Verification items for the finished model (mm, model axes). A direction names the side the tool comes from. Round coordinates to 2 decimals unless told otherwise and drop trailing zeros. Write each loop counter-clockwise with the first axis right and the second up, starting at its lowest first coordinate (ties: lowest second). Pieces come first, ordered by that corner, then holes. Notation, with made-up numbers: (-18, 33) - (-4, 33) arc R11 cw to (-4, 48) - close; hole circle Ø5 at (13.25, 3.25). An arc over 180 degrees is marked (long way). Answer as a JSON object with one key per item and string values.
```python
from build123d import *

# Parameters (mm, degrees)
F1_DEPTH = 50
F0_R     = 15
F2_DEPTH = 30
F3_R     = 10
F4_DEPTH = 42.2


with BuildPart() as f1:
    # F0 (on Front) → F1 (new body)
    with BuildSketch(Plane.XZ):
        with BuildLine():
            ThreePointArc((-4, -19.5959179423), (-12.6491106407, 15.4919333848), (20, 0))
            ThreePointArc((20, 0), (15.4919333848, -12.6491106407), (4, -19.5959179423))
            Line((4, -19.5959179423), (4, -25))
            Line((4, -25), (16.5831239518, -25))
            ThreePointArc((16.5831239518, -25), (20.3783390562, -22.0164324383), (23.6458608502, -18.4627534418))
            ThreePointArc((23.6458608502, -18.4627534418), (28.36702157, -9.7627909558), (30, 0))
            ThreePointArc((30, 0), (26.4338203685, 14.1863716546), (16.5831239518, 25))
            Line((16.5831239518, 25), (-16.5831239518, 25))
            ThreePointArc((-16.5831239518, 25), (-29.6115777819, 4.8119082768), (-23.6458608502, -18.4627534418))
            ThreePointArc((-23.6458608502, -18.4627534418), (-20.3783390562, -22.0164324383), (-16.5831239518, -25))
            Line((-16.5831239518, -25), (-4, -25))
            Line((-4, -25), (-4, -19.5959179423))
        make_face()
        with BuildLine():
            ThreePointArc((16.5831239518, 25), (0, 30), (-16.5831239518, 25))
            Line((-16.5831239518, 25), (16.5831239518, 25))
        make_face()
        with BuildLine():
            Line((16.5831239518, -57.5959179423), (16.5831239518, -25))
            ThreePointArc((16.5831239518, -25), (10.5600439971, -28.079983454), (4, -29.7321374946))
            Line((4, -29.7321374946), (4, -57.5959179423))
            Line((4, -57.5959179423), (16.5831239518, -57.5959179423))
        make_face()
        with BuildLine():
            Line((16.5831239518, -25), (4, -25))
            Line((4, -25), (4, -29.7321374946))
            ThreePointArc((4, -29.7321374946), (10.5600439971, -28.079983454), (16.5831239518, -25))
        make_face()
        with BuildLine():
            ThreePointArc((-4, -29.7321374946), (-10.5600439971, -28.079983454), (-16.5831239518, -25))
            Line((-16.5831239518, -25), (-16.5831239518, -57.5959179423))
            Line((-16.5831239518, -57.5959179423), (-4, -57.5959179423))
            Line((-4, -57.5959179423), (-4, -29.7321374946))
        make_face()
        with BuildLine():
            Line((-4, -29.7321374946), (-4, -25))
            Line((-4, -25), (-16.5831239518, -25))
            ThreePointArc((-16.5831239518, -25), (-10.5600439971, -28.079983454), (-4, -29.7321374946))
        make_face()
    extrude(amount=F1_DEPTH)

    # F0 (on Front) → F2 (join)
    with BuildSketch(Plane.XZ):
        with BuildLine():
            Line((-50, -25), (-23.6458608502, -18.4627534418))
            ThreePointArc((-23.6458608502, -18.4627534418), (-29.6115777819, 4.8119082768), (-16.5831239518, 25))
            Line((-16.5831239518, 25), (-85, 25))
            Line((-85, 25), (-85, -25))
            Line((-85, -25), (-50, -25))
        make_face()
        with Locations((-58.52034688, 0)):
            Circle(F0_R, mode=Mode.SUBTRACT)
        with BuildLine():
            ThreePointArc((30, 0), (28.36702157, -9.7627909558), (23.6458608502, -18.4627534418))
            Line((23.6458608502, -18.4627534418), (50, -25))
            Line((50, -25), (85, -25))
            Line((85, -25), (85, 25))
            Line((85, 25), (16.5831239518, 25))
            ThreePointArc((16.5831239518, 25), (26.4338203685, 14.1863716546), (30, 0))
        make_face()
        with Locations((58.52034688, 0)):
            Circle(F0_R, mode=Mode.SUBTRACT)
    extrude(amount=F2_DEPTH)

    # F3 (on face) → F4 (cut)
    with BuildSketch(Plane(origin=(-16.5831239518, 0, 0), x_dir=(0, -1, 0), z_dir=(-1, 0, 0))):
        with Locations((25, -43)):
            Circle(F3_R)
    extrude(amount=-F4_DEPTH, mode=Mode.SUBTRACT)


solid = f1.part
```
1. Material ranges on probe 1 along X at (y, z) = (-34, -35); probe 2 along X at (y, z) = (-32, 7) (3 decimals); probe 3 along Y at (x, z) = (-59.5, -19), recorded low to high. Write a range as from..to.
Completed:
{"probe 1": "x = -16.58..-4, 4..16.58", "probe 2": "x = -29.172..-18.735, 18.735..29.172", "probe 3": "y = -30..0"}
2. Cross-section at D-D (z = 7). Record the boundary of the cut face in (x, y) (3 decimals).
Completed:
{"outline": "(-85, -30) - (-71.787, -30) - (-71.787, 0) - (-85, 0) - close; (-45.254, -30) - (-29.172, -30) - (-29.172, -50) - (-18.735, -50) - (-18.735, 0) - (-45.254, 0) - close; (18.735, -50) - (29.172, -50) - (29.172, -30) - (45.254, -30) - (45.254, 0) - (18.735, 0) - close; (71.787, -30) - (85, -30) - (85, 0) - (71.787, 0) - close"}
3. Cross-section at C-C (x = 0). Record the boundary of the cut face in (y, z).
Completed:
{"outline": "(-50, 20) - (0, 20) - (0, 30) - (-50, 30) - close"}
4. Access from +Z, -Z, +X, -X, +Y, -Y to the whole of each face (thin tool, end or side, straight path). Record for faces 1 (the face through (-68, -15, -25)), 2 (the face through (-85, -15, 0)), 3 (the face through (16.583, -19, -34)), 4 (the face through (-37.007, -14.79, -21.777)), 5 (the face through (51, -15, 25)).
Completed:
{"face 1": "-Z, -X, +Y, -Y", "face 2": "+Z, -Z, -X, +Y, -Y", "face 3": "-Z, +X, +Y, -Y", "face 4": "-Z, +Y, -Y", "face 5": "+Z, +X, +Y, -Y"}
5. Go/stop test with flat-tipped pins: pin 1 (5 mm diameter, centred on y = -15, z = -34.5, fed in from +X); pin 2 (9 mm diameter, centred on x = -66, y = -21, fed in from -Z); pin 3 (12 mm diameter, centred on y = -40, z = 10.5, fed in from -X). Record where each tip stops, or that it passes through.
Completed:
{"pin 1": "stops at x = 16.58", "pin 2": "stops at z = -25", "pin 3": "stops at x = -29.66"}
6. Cross-section at A-A (y = -25). Record the boundary of the cut face in (x, z).
Completed:
{"outline": "(-85, -25) - (-50, -25) - (-23.65, -18.46) arc R30 ccw to (-16.58, -25) - (-16.58, -33) - (-4, -33) - (-4, -19.6) arc R20 cw (long way) to (4, -19.6) - (4, -33) - (16.58, -33) - (16.58, -25) arc R30 ccw to (23.65, -18.46) - (50, -25) - (85, -25) - (85, 25) - (16.58, 25) arc R30 ccw to (-16.58, 25) - (-85, 25) - close; (-16.58, -57.6) - (-4, -57.6) - (-4, -53) - (-16.58, -53) - close; (4, -57.6) - (16.58, -57.6) - (16.58, -53) - (4, -53) - close; hole circle Ø30 at (-58.52, 0); hole circle Ø30 at (58.52, 0)"}
7. Cross-section at B-B (z = -43). Record the boundary of the cut face in (x, y).
Completed:
{"outline": "(-16.58, -50) - (-4, -50) - (-4, -35) - (-16.58, -35) - close; (-16.58, -15) - (-4, -15) - (-4, 0) - (-16.58, 0) - close; (4, -50) - (16.58, -50) - (16.58, -35) - (4, -35) - close; (4, -15) - (16.58, -15) - (16.58, 0) - (4, 0) - close"}
8. Mould release check, pull along Z, two halves, no side actions. Record for faces 6 (the face through (43.535, -14.79, 0.66)), 7 (the face through (-50, -15, 25)), 8 (the face through (-44, -30, 6)), 9 (the face through (-70.42, -14.79, -9.13)): released by +Z, released by -Z, zero draft, split by the parting line, or undercut.
Completed:
{"face 6": "undercut", "face 7": "released by +Z", "face 8": "zero draft", "face 9": "undercut"}
